from build123d import *

# Parameters (mm, degrees)
SKETCH1_W           = 13.081
SKETCH1_H           = 8.128
SKETCH1_R           = 0.5
BOSS_EXTRUDE1_DEPTH = 1.3
SKETCH2_W           = 3
SKETCH2_H           = 3
BOSS_EXTRUDE2_DEPTH = 1.3
SKETCH3_W           = 1
SKETCH3_H           = 2.5
BOSS_EXTRUDE3_DEPTH = 1


with BuildPart() as part:
    # Sketch1 → Boss-Extrude1 (new body)
    with BuildSketch(Plane(origin=(0, 0, 0), x_dir=(1, 0, 0), z_dir=(0, 1, 0))):
        Rectangle(SKETCH1_W, SKETCH1_H)
        with Locations(Location((-5.0405, 2.54, 0), (0, 0, 270))):
            Circle(SKETCH1_R, mode=Mode.SUBTRACT)
        with Locations(Location((-5.0405, 0, 0), (0, 0, 270))):
            Circle(SKETCH1_R, mode=Mode.SUBTRACT)
        with Locations(Location((-5.0405, -2.54, 0), (0, 0, 270))):
            Circle(SKETCH1_R, mode=Mode.SUBTRACT)
    extrude(amount=BOSS_EXTRUDE1_DEPTH)

    # Sketch2 → Boss-Extrude2 (add)
    with BuildSketch(Plane(origin=(0, 1.3, 0), x_dir=(1, 0, 0), z_dir=(0, 1, 0))):
        with Locations((2.0405, -1.564)):
            Rectangle(SKETCH2_W, SKETCH2_H)
    extrude(amount=BOSS_EXTRUDE2_DEPTH)

    # Sketch3 → Boss-Extrude3 (add)
    with BuildSketch(Plane(origin=(0, 1.3, 0), x_dir=(1, 0, 0), z_dir=(0, 1, 0))):
        with Locations((2.0405, 1.814)):
            Rectangle(SKETCH3_W, SKETCH3_H)
    extrude(amount=BOSS_EXTRUDE3_DEPTH)


solid = part.part
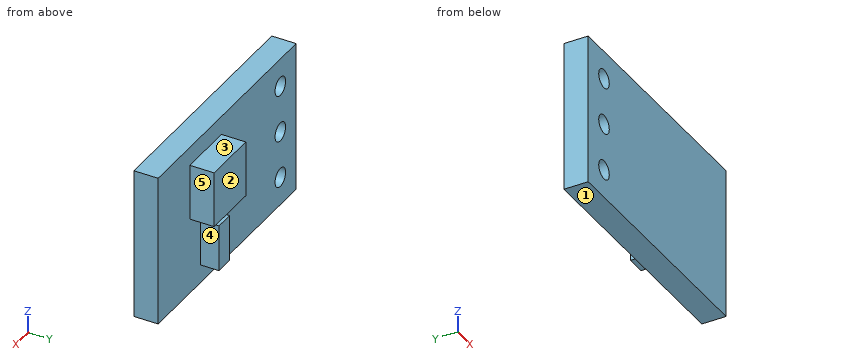
Part model, mm, in its own coordinate system. Face numbers are marked on the shaded views. A direction names the side the tool comes from. Give positions to 0.01 mm unless a question says otherwise; leave off trailing zeros. Order: outer loops, then holes, each group sorted by start corner. A loop starts at its lowest first (then second) coordinate and runs counter-clockwise, first axis right, second up. Notation, with made-up numbers: (26, 67) -> (45, 67) arc R19 cw to (45, 87) -> close; hole circle Ø2 at (10.25, 13). An arc over 180 degrees is marked (long way). Use one line per item in the form item = value.
(1) Saw through at A-A (z = 2.54). Write the cut outline in (x, y), then the cut area to 3 significant figures.
Solution:
outline = (-6.54, 0) -> (-5.54, 0) -> (-5.54, 1.3) -> (-6.54, 1.3) -> close; (-4.54, 0) -> (6.54, 0) -> (6.54, 1.3) -> (3.54, 1.3) -> (3.54, 2.6) -> (0.54, 2.6) -> (0.54, 1.3) -> (-4.54, 1.3) -> close
area = 19.6 mm²
(2) Tool access for the marked faces 1, 2, 3, 4 and 5: list every direction of +Z, -Z, +X, -X, +Y, -Y with a clear straight run to the whole face (end or side of a thin tool).
Solution:
face_1 = -Z, +X, -X, +Y, -Y
face_2 = +Z, -Z, +X, -X, +Y
face_3 = +Z, +X, -X, +Y
face_4 = -Z, +X, +Y
face_5 = +Z, -Z, +X, +Y
(3) Saw through at B-B (y = 2.1). Write the cut outline in (x, z).
Solution:
outline = (0.54, 0.06) -> (3.54, 0.06) -> (3.54, 3.06) -> (0.54, 3.06) -> close; (1.54, -3.06) -> (2.54, -3.06) -> (2.54, -0.56) -> (1.54, -0.56) -> close
(4) Drill centre lines: line 1 (X direction, y = 0.3, z = 2.54); line 2 (Y direction, x = -5, z = -1); line 3 (X direction, y = 1.9, z = 3). Where is each one in solid material? Low to high. Write a range as from..to.
Solution:
line_1 = -6.54..-5.54, -4.54..6.54
line_2 = 0..1.3
line_3 = 0.54..3.54
(5) Flat gauge pins, fed straight in: P1, Ø3, axis at x = 2, z = 0.5, coming from the -Y side; P2, Ø0.5, axis at x = 2, y = 2, coming from the -Z side; P3, Ø1, axis at x = 2, y = 2, coming from the +Z side. Where does each tip first touch, or does it go through?
Solution:
P1 = 0
P2 = -3.06
P3 = 3.06
(6) Saw through at D-D (x = -4.75). Write the cut outline in (y, z).
Solution:
outline = (0, -4.06) -> (1.3, -4.06) -> (1.3, -2.95) -> (0, -2.95) -> close; (0, -2.13) -> (1.3, -2.13) -> (1.3, -0.41) -> (0, -0.41) -> close; (0, 0.41) -> (1.3, 0.41) -> (1.3, 2.13) -> (0, 2.13) -> close; (0, 2.95) -> (1.3, 2.95) -> (1.3, 4.06) -> (0, 4.06) -> close
(7) Saw through at C-C (z = 1.5). Write the cut outline in (x, y), then the cut area to 3 significant figures.
Solution:
outline = (-6.54, 0) -> (6.54, 0) -> (6.54, 1.3) -> (3.54, 1.3) -> (3.54, 2.6) -> (0.54, 2.6) -> (0.54, 1.3) -> (-6.54, 1.3) -> close
area = 20.9 mm²
